For this review, take the finished solid that the model builds, in its own axes (mm). Face numbers are marked on the shaded views. Give positions to 0.01 mm unless a question says otherwise; leave off trailing zeros. Loops run counter-clockwise (first coordinate to the right, second up) from the corner with the lowest first, then second, coordinate; pieces in that order, holes last.
Autodesk Inventor part; units mm, degrees
ref_plane "YZ Plane" through (0, 0, 0) normal (1, 0, 0) x (0, 1, 0)
ref_plane "XZ Plane" through (0, 0, 0) normal (0, 1, 0) x (-1, 0, 0)
ref_plane "XY Plane" through (0, 0, 0) normal (0, 0, 1) x (1, 0, 0)
ref_plane "Work Plane1" through (0, 0, -2) normal (0, 0, 1) x (-1, 0, 0)
sketch "Sketch1" plane through (0, 0, -2) normal (0, 0, 1) x (-1, 0, 0)
  circle A0 centre (0, 0) radius 8.1117
  circle A1 centre (0, 0) radius 8.3117
  circle A2 centre (0, 0) radius 9.1117
  point P0 (0, 0)
  dimension "d0" = 0.2
  dimension "d1" = 1
extrude "Extrusion1" add sketch "Sketch1" against normal blind 10 contours A2
sketch "Sketch2" plane through (0, 0, -2) normal (0, 0, 1) x (1, 0, 0)
  circle A0 centre (0, 0) radius 8.3117
  circle A1 centre (0, 0) radius 9.6318
  point P0 (0, 0)
extrude "Extrusion2" add sketch "Sketch2" along normal blind 0.5
sketch "Sketch3" plane through (0, 0, -12) normal (0, 0, -1) x (-1, 0, 0)
  circle A0 centre (0, 0) radius 9.6318
  circle A1 centre (0, 0) radius 8.3117
  point P0 (0, 0)
extrude "Extrusion3" add sketch "Sketch3" along normal blind 0.5
properties part number "01_Autofocus_10x_objective_copper_coil"
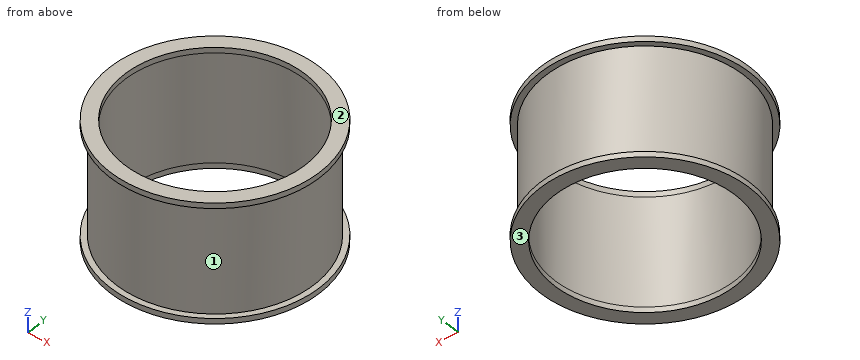
Q1. For probe 1 along X at (y, z) = (0, -8); probe 2 along Y at (x, z) = (0, -1.7); probe 3 along Z at (x, y) = (-8.25, 4.75), list the stretches that pass through material, from the lowest coordinate up.
Answers:
probe 1: x = -9.11 to -8.31, 8.31 to 9.11
probe 2: y = -9.63 to -8.31, 8.31 to 9.63
probe 3: z = -12.5 to -12, -2 to -1.5
Q2. For pin 1 Ø2 at (x, z) = (-2, -5) entering from -Y; pin 2 Ø1.5 at (y, z) = (-4.5, -10.5) entering from -X; pin 3 Ø9.5 at (x, y) = (-1, -3) entering from -Z; pin 4 Ø2 at (x, z) = (-6.5, -9.5) entering from -Y, all flat-tipped, find the tip position at first contact; note any pin that passes through.
Answers:
pin 1: stops at y = -9.06
pin 2: stops at x = -8.3
pin 3: passes through
pin 4: stops at y = -7.26
Q3. Consider section C-C on z = -2.5. Give the boundary of the cut face in (x, y).
Answers:
outline: circle Ø18.22 at (0, 0); hole circle Ø16.62 at (0, 0)
Q4. Mouldability with a two-part tool opening along Z and no side actions: class the marked faces 1, 2 and 3 as +Z half, -Z half, draft (parallel to the pull), parting line (faces both ways), or undercut.
Answers:
face 1: undercut
face 2: +Z half
face 3: -Z half
Q5. Consider section B-B on y = -5.75. Give the boundary of the cut face in (x, z).
Answers:
outline: (-7.73, -12.5) - (-6, -12.5) - (-6, -1.5) - (-7.73, -1.5) - (-7.73, -2) - (-7.07, -2) - (-7.07, -12) - (-7.73, -12) - close; (6, -12.5) - (7.73, -12.5) - (7.73, -12) - (7.07, -12) - (7.07, -2) - (7.73, -2) - (7.73, -1.5) - (6, -1.5) - close
Q6. Consider section A-A on x = 0. Give the boundary of the cut face in (y, z).
Answers:
outline: (-9.63, -12.5) - (-8.31, -12.5) - (-8.31, -1.5) - (-9.63, -1.5) - (-9.63, -2) - (-9.11, -2) - (-9.11, -12) - (-9.63, -12) - close; (8.31, -12.5) - (9.63, -12.5) - (9.63, -12) - (9.11, -12) - (9.11, -2) - (9.63, -2) - (9.63, -1.5) - (8.31, -1.5) - close
